The listing builds one solid part. Answer for the finished solid, in the listing's coordinates (mm). Face numbers are marked on the shaded views. Round coordinates to 2 decimals unless told otherwise and drop trailing zeros. Write each loop counter-clockwise with the first axis right and the second up, starting at its lowest first coordinate (ties: lowest second). Pieces come first, ordered by that corner, then holes.
from build123d import *

# Parameters (mm, degrees)
SKETCH1_R                       = 40
SKETCH1_R_2                     = 30
BOSS_EXTRUDE1_DEPTH             = 10
M4X0_7_TAPPED_HOLE1_D           = 3.3
M4X0_7_TAPPED_HOLE1_CSINK_D     = 4.05
M4X0_7_TAPPED_HOLE1_CSINK_ANGLE = 90
CIRPATTERN1_COUNT               = 6
SKETCH14_R                      = 25
BOSS_EXTRUDE5_DEPTH             = 10
BOSS_EXTRUDE7_START             = 10
SKETCH15_W                      = 7.5
SKETCH15_H                      = 15
SKETCH15_R                      = 2.025
BOSS_EXTRUDE7_DEPTH             = 10


with BuildPart() as part:
    # Sketch1 → Boss-Extrude1 (new body)
    with BuildSketch(Plane.XY):
        Circle(SKETCH1_R)
        Circle(SKETCH1_R_2, mode=Mode.SUBTRACT)
    extrude(amount=-BOSS_EXTRUDE1_DEPTH)

    # M4x0.7 Tapped Hole1 (through all)
    with Locations(Plane.XY):
        with Locations((36.25, 0)):
            m4x0_7_tapped_hole1 = CounterSinkHole(M4X0_7_TAPPED_HOLE1_D / 2, M4X0_7_TAPPED_HOLE1_CSINK_D / 2, counter_sink_angle=M4X0_7_TAPPED_HOLE1_CSINK_ANGLE)

    # CirPattern1: M4x0.7 Tapped Hole1 ×6 about axis
    cirpattern1_axis = Axis((0, 0, 0), (0, 0, 1))
    for i in range(1, CIRPATTERN1_COUNT):
        add(m4x0_7_tapped_hole1.rotate(cirpattern1_axis, i * 360 / CIRPATTERN1_COUNT), mode=Mode.SUBTRACT)

    # Sketch14 → Boss-Extrude5 (add)
    with BuildSketch(Plane.XY):
        with BuildLine():
            ThreePointArc((39.949968711, -2), (0, -40), (-39.949968711, -2))
            Line((-39.949968711, -2), (-24.968730444, -301.25))
            ThreePointArc((-24.968730444, -301.25), (-0.625195526, -275.007818612), (25, -300))
            ThreePointArc((25, -300), (24.992181388, -300.625195526), (24.968730444, -301.25))
            Line((24.968730444, -301.25), (39.949968711, -2))
        make_face()
        with Locations((0, -300)):
            Circle(SKETCH14_R)
    extrude(amount=-BOSS_EXTRUDE5_DEPTH)

    # Sketch15 → Boss-Extrude7 (add)
    # profile 1 of 4: a face of its own
    with BuildSketch(Plane.XY.offset(BOSS_EXTRUDE7_START)):
        with Locations((3.75, -232.5)):
            Rectangle(SKETCH15_W, SKETCH15_H)
    # profile 2 of 4: a face of its own
    with BuildSketch(Plane.XY.offset(BOSS_EXTRUDE7_START)):
        with Locations((-3.75, -232.5)):
            Rectangle(SKETCH15_W, SKETCH15_H)
    # profile 3 of 4: a face of its own
    with BuildSketch(Plane.XY.offset(BOSS_EXTRUDE7_START)):
        with BuildLine():
            Line((20.390984754, -192.690398552), (30.40350824, -192.690398552))
            Line((30.40350824, -192.690398552), (39.949968711, -2))
            ThreePointArc((39.949968711, -2), (28.982753492, 27.568097504), (0, 40))
            Line((0, 40), (0, 30))
            ThreePointArc((0, 30), (21.213203436, 21.213203436), (30, 0))
            ThreePointArc((30, 0), (24.494897428, -17.320508076), (10, -28.284271247))
            Line((10, -28.284271247), (10, -38.284271247))
            Line((10, -38.284271247), (27.650064281, -47.690398552))
            Line((27.650064281, -47.690398552), (20.390984754, -192.690398552))
        make_face()
        with Locations((18.125, -31.393420887)):
            Circle(SKETCH15_R, mode=Mode.SUBTRACT)
        with Locations((18.125, 31.393420887)):
            Circle(SKETCH15_R, mode=Mode.SUBTRACT)
        with Locations((36.25, 0)):
            Circle(SKETCH15_R, mode=Mode.SUBTRACT)
    # profile 4 of 4: a face of its own
    with BuildSketch(Plane.XY.offset(BOSS_EXTRUDE7_START)):
        with BuildLine():
            Line((-39.949968711, -2), (-30.40350824, -192.690398552))
            Line((-30.40350824, -192.690398552), (-20.390984754, -192.690398552))
            Line((-20.390984754, -192.690398552), (-27.650064281, -47.690398552))
            Line((-27.650064281, -47.690398552), (-10, -38.284271247))
            Line((-10, -38.284271247), (-10, -28.284271247))
            ThreePointArc((-10, -28.284271247), (-29.56795679, 5.073059362), (0, 30))
            Line((0, 30), (0, 40))
            ThreePointArc((0, 40), (-28.982753492, 27.568097504), (-39.949968711, -2))
        make_face()
        with Locations((-36.25, 0)):
            Circle(SKETCH15_R, mode=Mode.SUBTRACT)
        with Locations((-18.125, -31.393420887)):
            Circle(SKETCH15_R, mode=Mode.SUBTRACT)
        with Locations((-18.125, 31.393420887)):
            Circle(SKETCH15_R, mode=Mode.SUBTRACT)
    extrude(amount=-BOSS_EXTRUDE7_DEPTH)


solid = part.part
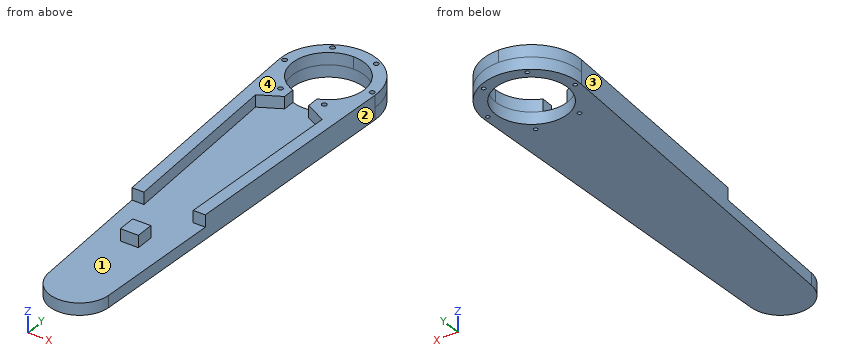
1. For a pull along X with two mould halves and no side action, classify the marked faces 1, 2, 3 and 4 as released by +X, released by -X, zero draft, split by the parting line, or undercut.
Geometry says:
face 1: undercut
face 2: released by +X
face 3: released by -X
face 4: zero draft
2. Section C-C on y = -112.5 is taken. Determine the outline of the cut face in (x, z).
Geometry says:
outline: (-34.42, -10) - (34.42, -10) - (34.42, 10) - (24.41, 10) - (24.41, 0) - (-24.41, 0) - (-24.41, 10) - (-34.42, 10) - close
3. Straight lines are drawn through the part: line 1 along Z through (x, y) = (-17.5, -128); line 2 along X through (y, z) = (-90.5, 4.25); line 3 along Y through (x, z) = (-20.5, -4). For each, find the intervals that lie inside material, in ascending order.
Geometry says:
line 1: z = -10 to 0
line 2: x = -35.52 to -25.51, 25.51 to 35.52
line 3: y = -314.31 to -21.9, 21.9 to 34.35
4. Given pin 1 (11 mm diameter, centred on y = -232.5, z = 4.5, fed in from +X); pin 2 (6 mm diameter, centred on x = -25, z = 7, fed in from -Y); pin 3 (6 mm diameter, centred on x = -18, y = -85, fed in from +Z), each flat-ended and moving along its own axis, determine where each tip first touches the part or whether it passes through.
Geometry says:
pin 1: stops at x = 28.57
pin 2: stops at y = -192.69
pin 3: stops at z = 0
5. Section A-A on z = -4.25 is taken. Determine the outline of the cut face in (x, y) (3 decimals).
Geometry says:
outline: (-39.95, -2) - (-24.969, -301.25) arc R25 ccw to (24.969, -301.25) - (39.95, -2) arc R40 ccw (long way) to start; hole circle Ø3.3 at (-36.25, 0); hole circle Ø60 at (0, 0); hole circle Ø3.3 at (-18.125, -31.393); hole circle Ø3.3 at (-18.125, 31.393); hole circle Ø3.3 at (18.125, -31.393); hole circle Ø3.3 at (18.125, 31.393); hole circle Ø3.3 at (36.25, 0)
6. Section B-B on y = -188 is taken. Determine the outline of the cut face in (x, z).
Geometry says:
outline: (-30.64, -10) - (30.64, -10) - (30.64, 10) - (20.63, 10) - (20.63, 0) - (-20.63, 0) - (-20.63, 10) - (-30.64, 10) - close
